Design review of the part built by this model. Coordinates are the model's own, in mm. A direction names the side the tool comes from. Coordinates: 2 decimals unless noted, no trailing zeros. Loops run counter-clockwise (first coordinate to the right, second up) from the corner with the lowest first, then second, coordinate; pieces in that order, holes last. Notation, with made-up numbers: (45, 73.5) -> (53, 73.5) arc R22 cw to (53, 102.5) -> close; hole circle Ø7 at (89, 50.5). An arc over 180 degrees is marked (long way). Answer as a JSON object with one key per item and string values.
```python
from build123d import *

# Parameters (mm, degrees)
SKETCH1_W           = 31
SKETCH1_H           = 14
BOSS_EXTRUDE1_DEPTH = 1
SKETCH2_W           = 4
SKETCH2_H           = 4
BOSS_EXTRUDE2_DEPTH = 10
SKETCH3_R           = 1.5
CUT_EXTRUDE1_DEPTH  = 36.454195802
SKETCH4_W           = 4
SKETCH4_H           = 5
BOSS_EXTRUDE3_DEPTH = 2.5
SKETCH_1_W          = 1.2
SKETCH_1_H          = 10
EXTRUDE_1_DEPTH     = 1.2
SKETCH_2_W          = 0.519767639
SKETCH_2_H          = 0.519767639
SKETCH_2_H_2        = 0.580916774
SKETCH_2_H_3        = 0.550342206
SKETCH_2_H_4        = 0.61149134
EXTRUDE_2_DEPTH     = 1
SKETCH_3_W          = 0.61149134
SKETCH_3_H          = 0.60685635
SKETCH_3_W_2        = 0.550342206
SKETCH_3_W_3        = 0.580916774
SKETCH_3_W_4        = 0.519767639
EXTRUDE_3_DEPTH     = 10


with BuildPart() as part:
    # Sketch1 → Boss-Extrude1 (new body)
    with BuildSketch(Plane(origin=(0, 0, 0), x_dir=(1, 0, 0), z_dir=(0, 1, 0))):
        with Locations((15.5, -7)):
            Rectangle(SKETCH1_W, SKETCH1_H)
    extrude(amount=BOSS_EXTRUDE1_DEPTH)

    # Sketch2 → Boss-Extrude2 (add)
    with BuildSketch(Plane(origin=(0, 1, 0), x_dir=(1, 0, 0), z_dir=(0, 1, 0))):
        with Locations((4, -11.5)):
            Rectangle(SKETCH2_W, SKETCH2_H)
        with Locations((4, -2.5)):
            Rectangle(SKETCH2_W, SKETCH2_H)
    extrude(amount=BOSS_EXTRUDE2_DEPTH)

    # Sketch3 → Cut-Extrude1 (cut, through all)
    with BuildSketch(Plane(origin=(0, 1, 0), x_dir=(1, 0, 0), z_dir=(0, 1, 0))):
        with Locations(Location((26, -7, 0), (0, 0, 270))):
            Circle(SKETCH3_R)
    extrude(amount=-CUT_EXTRUDE1_DEPTH, mode=Mode.SUBTRACT)

    # Sketch4 → Boss-Extrude3 (add)
    with BuildSketch(Plane(origin=(0, 1, 0), x_dir=(1, 0, 0), z_dir=(0, 1, 0))):
        with Locations((4, -7)):
            Rectangle(SKETCH4_W, SKETCH4_H)
    extrude(amount=BOSS_EXTRUDE3_DEPTH)

    # 草图1 → 凸台-拉伸1 (add)
    with BuildSketch(Plane(origin=(0, 1, 0), x_dir=(1, 0, 0), z_dir=(0, 1, 0))):
        with Locations((30.150896117, -7)):
            Rectangle(SKETCH_1_W, SKETCH_1_H)
    extrude(amount=EXTRUDE_1_DEPTH)

    # 草图2 → 凸台-拉伸2 (add)
    with BuildSketch(Plane(origin=(0, 2.2, 0), x_dir=(1, 0, 0), z_dir=(0, 1, 0))):
        with Locations((30.20363542, -3.636797628)):
            Rectangle(SKETCH_2_W, SKETCH_2_H)
        with Locations((30.20363542, -5.685293618)):
            Rectangle(SKETCH_2_W, SKETCH_2_H_2)
        with Locations((30.20363542, -8.024247995)):
            Rectangle(SKETCH_2_W, SKETCH_2_H_3)
        with Locations((30.20363542, -10.225616821)):
            Rectangle(SKETCH_2_W, SKETCH_2_H_4)
    extrude(amount=EXTRUDE_2_DEPTH)

    # 草图3 → 凸台-拉伸3 (add)
    with BuildSketch(Plane(origin=(30.463519239, 0, 0), x_dir=(0, 0, -1), z_dir=(1, 0, 0))):
        with Locations((-10.225616821, 2.896571825)):
            Rectangle(SKETCH_3_W, SKETCH_3_H)
        with Locations((-8.024247995, 2.896571825)):
            Rectangle(SKETCH_3_W_2, SKETCH_3_H)
        with Locations((-5.685293618, 2.896571825)):
            Rectangle(SKETCH_3_W_3, SKETCH_3_H)
        with Locations((-3.636797628, 2.896571825)):
            Rectangle(SKETCH_3_W_4, SKETCH_3_H)
    extrude(amount=EXTRUDE_3_DEPTH)


solid = part.part
```
1) Add section A-A, the plane z = 7. Give the boundary of the cut face in (x, y), and give its area (3 significant figures).
Completed:
{"outline": "(0, 0) -> (24.5, 0) -> (24.5, 1) -> (6, 1) -> (6, 3.5) -> (2, 3.5) -> (2, 1) -> (0, 1) -> close; (27.5, 0) -> (31, 0) -> (31, 1) -> (30.75, 1) -> (30.75, 2.2) -> (29.55, 2.2) -> (29.55, 1) -> (27.5, 1) -> close", "area": "39.4 mm²"}
2) Add section D-D, the plane x = 26. Give the boundary of the cut face in (y, z).
Completed:
{"outline": "(0, 0) -> (1, 0) -> (1, 5.5) -> (0, 5.5) -> close; (0, 8.5) -> (1, 8.5) -> (1, 14) -> (0, 14) -> close"}
3) Wall thickness on probe 1 along X at (y, z) = (0.3, 7); probe 2 along X at (y, z) = (1.5, 8.25); probe 3 along X at (y, z) = (3.5, 9.75): over which ranges is each line inside the solid? List them lowest first.
Completed:
{"probe 1": "0 to 24.5, 27.5 to 31", "probe 2": "2 to 6, 29.55 to 30.75", "probe 3": "2 to 6"}
4) Clearance check with flat-ended pins moving along their axes: pin 1 Ø5 at (x, z) = (24.5, 2) entering from -Y; pin 2 Ø3 at (x, y) = (4.5, 8) entering from -Z; pin 3 Ø2 at (y, z) = (8, 2) entering from -X; pin 4 Ø0.5 at (x, y) = (33, 2.5) entering from -Z. State where each tip first meets the part, or that it passes through.
Completed:
{"pin 1": "y = 0", "pin 2": "z = 0.5", "pin 3": "x = 2", "pin 4": "z = 3.38"}
5) For faces 5 (the flat face through (30.751, 2, 7)), 6 (the flat face through (4, 3.5, 7)), 7 (the flat face through (30, 2, 2)), list the 3-axis set-ups (+Z, -Z, +X, -X, +Y, -Y) from which the entire face can be reached by the end or side of a thin tool; tool diameter is ignored.
Completed:
{"face 5": "+Z, -Z, +X", "face 6": "+X, -X, +Y", "face 7": "-Z, +X, +Y"}
6) The part is to be moulded in two halves that separate along Z. For faces 1 (the flat face through (30, 2, 12)), 2 (the flat face through (35, 3, 9.92)), 3 (the flat face through (4, 6, 0.5)), 4 (the flat face through (35, 3, 7.749)), say which applies: pulls with the +Z half, pulls with the -Z half, needs draft (parallel to the pull), parting line crosses it, or undercut.
Completed:
{"face 1": "pulls with the +Z half", "face 2": "undercut", "face 3": "pulls with the -Z half", "face 4": "undercut"}
7) Add section C-C, the plane y = 10. Give the boundary of the cut face in (x, z).
Completed:
{"outline": "(2, 0.5) -> (6, 0.5) -> (6, 4.5) -> (2, 4.5) -> close; (2, 9.5) -> (6, 9.5) -> (6, 13.5) -> (2, 13.5) -> close"}
8) Add section B-B, the plane x = 32.5. Give the boundary of the cut face in (y, z).
Completed:
{"outline": "(2.59, 3.38) -> (3.2, 3.38) -> (3.2, 3.9) -> (2.59, 3.9) -> close; (2.59, 5.39) -> (3.2, 5.39) -> (3.2, 5.98) -> (2.59, 5.98) -> close; (2.59, 7.75) -> (3.2, 7.75) -> (3.2, 8.3) -> (2.59, 8.3) -> close; (2.59, 9.92) -> (3.2, 9.92) -> (3.2, 10.53) -> (2.59, 10.53) -> close"}
